Can you work these out from the model? Positions are in its coordinate system, mm. Give positions to 0.01 mm unless a question says otherwise; leave off trailing zeros. Loops run counter-clockwise (first coordinate to the right, second up) from the corner with the lowest first, then second, coordinate; pieces in that order, holes last. Notation, with made-up numbers: M -16.5,81 L -4.5,81 A22 cw -4.5,99 Z; hole C 53.5,-25.75 d1. An arc over 180 degrees is marked long. Use CSV: the item, a comma, the result in double quotes.
Autodesk Inventor part; units mm, degrees
ref_plane "YZ Plane" through (0, 0, 0) normal (1, 0, 0) x (0, 1, 0)
ref_plane "XZ Plane" through (0, 0, 0) normal (0, 1, 0) x (-1, 0, 0)
ref_plane "XY Plane" through (0, 0, 0) normal (0, 0, 1) x (1, 0, 0)
sketch "Sketch1" plane through (0, 0, 0) normal (0, 0, 1) x (1, 0, 0)
  line L0 (-73.2051, 41.2219) -> (-136.7051, 41.2219)
  line L1 (-143.0551, 47.5719) -> (-143.0551, 98.3719)
  line L2 (-143.0551, 98.3719) -> (-66.8551, 98.3719)
  line L3 (-66.8551, 98.3719) -> (-66.8551, 47.5719)
  line L4 (-143.0551, 47.5719) -> (-136.7051, 41.2219)
  line L5 (-73.2051, 41.2219) -> (-66.8551, 47.5719)
  point P0 (0, 0)
  point P1 (-66.8551, 41.2219)
  point P2 (-143.0551, 41.2219)
  point P3 (-117.6551, 41.2219)
  point P4 (-143.0551, 66.6219)
  point P5 (-66.8551, 72.9719)
  point P6 (-92.2551, 41.2219)
  point P7 (-143.0551, 41.2219)
  point P8 (-66.8551, 41.2219)
  dimension "d0" = 76.2
  dimension "d1" = 57.15
  dimension "d10" = 6.35
  dimension "d11" = 6.35
  dimension "d12" = 6.35
extrude "Extrusion1" add sketch "Sketch1" along normal blind 6.35
sketch "Sketch2" plane through (0, 0, 6.35) normal (0, 0, 1) x (1, 0, 0)
  line L0 (-130.3551, 77.0986) -> (-130.3551, 56.1453)
  line L1 (-130.3551, 66.6219) -> (-98.3601, 66.6219) construction
  arc A0 (-119.7326, 65.7975) -> (-124.4934, 65.9243) centre (-122.0928, 66.6219) ccw
  line L2 (-124.4934, 65.9243) -> (-119.7326, 65.7975)
  point P0 (0, 0)
  dimension "d4" = 5
extrude "Extrusion2" cut sketch "Sketch2" against normal through all
sketch "Sketch3" plane through (0, 0, 0) normal (0, 0, -1) x (-1, 0, 0)
  arc A0 (124.4934, 65.9243) -> (119.7326, 65.7975) centre (122.0928, 66.6219) ccw
  line L0 (124.4934, 65.9243) -> (119.7326, 65.7975)
  circle A1 centre (122.0928, 66.6219) radius 11
  point P0 (0, 0)
extrude "Extrusion3" cut sketch "Sketch3" against normal through all
sketch "Sketch4" plane through (0, 0, 0) normal (0, 0, -1) x (-1, 0, 0)
  line L0 (143.0551, 92.0219) -> (133.3409, 92.0219) construction
  line L1 (143.0551, 85.6719) -> (133.3409, 85.6719) construction
  line L2 (143.0551, 85.6719) -> (143.0551, 98.3719) construction
  line L3 (35.1051, 88.8469) -> (143.0551, 88.8469) construction
  circle A0 centre (77.2251, 88.8469) radius 1.8542
  circle A1 centre (131.4867, 88.8469) radius 1.8542
  line L4 (133.3409, 92.0219) -> (133.3409, 85.6719)
  point P0 (0, 0)
  dimension "d15" = 3.7084
  dimension "d16" = 3.7084
extrude "Extrusion4" cut sketch "Sketch4" against normal through all
properties part number "projectorMountSide" material "Nylon, molybdenum disulphide"
Q1. I want a section at B-B, the plane y = 58.5. Please give me the cut outline in (x, z), then the cut area to 3 significant figures.
Model answer:
outline,"M -143.06,0 L -129.51,0 L -129.51,6.35 L -143.06,6.35 Z; M -114.67,0 L -66.86,0 L -66.86,6.35 L -114.67,6.35 Z"
area,"390 mm2"
Q2. Please list where these lines run through material, in increasing order: L1, parallel to Y at x = -77, z = 6; L2, parallel to Y at x = -131, z = 1.5; L3, parallel to X at y = 88.5, z = 1.75. Write a range as from..to.
Model answer:
L1,"41.22..87.01, 90.69..98.37"
L2,"41.22..60.17, 73.08..87.06, 90.64..98.37"
L3,"-143.06..-133.31, -129.67..-79.05, -75.4..-66.86"
Q3. I want a section at C-C, the plane z = 1.5. Please give me the cut outline in (x, y).
Model answer:
outline,"M -143.06,47.57 L -136.71,41.22 L -73.21,41.22 L -66.86,47.57 L -66.86,98.37 L -143.06,98.37 Z; hole C -131.49,88.85 d3.71; hole C -122.09,66.62 d22; hole C -77.23,88.85 d3.71"
Q4. I'm going to push a flat-ended pin straight in: P1, Ø8, axis at x = -133, y = 84.5, coming from the -Z side. Where does the tip first touch, or does it pass through?
Model answer:
P1,"z = 0"
Q5. If we mould it in two halves opening along X, with no side actions, what happens to faces 1 (the flat face through (-105, 70, 6.35)), 2 (the cylindrical face through (-132.34, 87.2, 3.13)), 3 (the flat face through (-143.055, 73, 3))? For each: released by +X, released by -X, zero draft, split by the parting line, or undercut.
Model answer:
face 1,"zero draft"
face 2,"undercut"
face 3,"released by -X"
Q6. I want a section at A-A, the plane x = -121. Please give me the cut outline in (y, z).
Model answer:
outline,"M 41.22,0 L 55.68,0 L 55.68,6.35 L 41.22,6.35 Z; M 77.57,0 L 98.37,0 L 98.37,6.35 L 77.57,6.35 Z"
